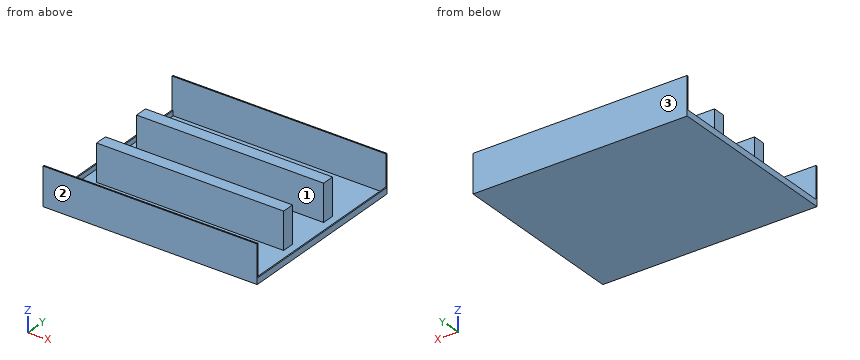
from build123d import *

# Parameters (mm, degrees)
SZKIC1_W                    = 172
SZKIC1_H                    = 144
DODANIE_WYCI_GNI_CIE1_DEPTH = 1
SZKIC1_3_W                  = 174
SZKIC1_3_H                  = 146
SZKIC1_3_W_2                = 172
SZKIC1_3_H_2                = 144
DODANIE_WYCI_GNI_CIE2_DEPTH = 5
SZKIC2_W                    = 152
SZKIC2_H                    = 10
DODANIE_WYCI_GNI_CIE4_DEPTH = 30
SZKIC4_W                    = 174
SZKIC4_H                    = 1
DODANIE_WYCI_GNI_CIE5_DEPTH = 26


with BuildPart() as part:
    # Szkic1 → Dodanie-wyciągnięcie1 (new body)
    with BuildSketch(Plane.XY):
        with Locations((86, 72)):
            Rectangle(SZKIC1_W, SZKIC1_H)
    extrude(amount=DODANIE_WYCI_GNI_CIE1_DEPTH)

    # Szkic1<3> → Dodanie-wyciągnięcie2 (add)
    with BuildSketch(Plane.XY):
        with Locations((86, 72)):
            Rectangle(SZKIC1_3_W, SZKIC1_3_H)
        with Locations((86, 72)):
            Rectangle(SZKIC1_3_W_2, SZKIC1_3_H_2, mode=Mode.SUBTRACT)
    extrude(amount=DODANIE_WYCI_GNI_CIE2_DEPTH)

    # Szkic2 → Dodanie-wyciągnięcie4 (add)
    with BuildSketch(Plane.XY.offset(1)):
        with Locations((86, 49)):
            Rectangle(SZKIC2_W, SZKIC2_H)
        with Locations((86, 94)):
            Rectangle(SZKIC2_W, SZKIC2_H)
    extrude(amount=DODANIE_WYCI_GNI_CIE4_DEPTH)

    # Szkic4 → Dodanie-wyciągnięcie5 (add)
    with BuildSketch(Plane.XY.offset(5)):
        with Locations((86, -0.5)):
            Rectangle(SZKIC4_W, SZKIC4_H)
        with Locations((86, 144.5)):
            Rectangle(SZKIC4_W, SZKIC4_H)
    extrude(amount=DODANIE_WYCI_GNI_CIE5_DEPTH)


solid = part.part
Work out the finished part from the listing and answer in its coordinate system (mm). Face numbers are marked on the shaded views. Give positions to 0.01 mm unless a question says otherwise; leave off trailing zeros. Order: outer loops, then holes, each group sorted by start corner. A loop starts at its lowest first (then second) coordinate and runs counter-clockwise, first axis right, second up. Notation, with made-up numbers: M 66.5,-6 L 86.5,-6 A26 ccw 86.5,27 Z; hole C -33.5,-26.5 d6. An arc over 180 degrees is marked long. Return JSON: item names as keys, results as strings.
Q1. Find section A-A, the plane z = 8.5. Write down the section's boundary in (x, y), and give its area (3 significant figures).
Answer below:
{"outline": "M -1,-1 L 173,-1 L 173,0 L -1,0 Z; M -1,144 L 173,144 L 173,145 L -1,145 Z; M 10,44 L 162,44 L 162,54 L 10,54 Z; M 10,89 L 162,89 L 162,99 L 10,99 Z", "area": "3,390 mm^2"}
Q2. The mould has two halves that part along Y. Classify the marked faces 1, 2 and 3: pulls with the +Y half, pulls with the -Y half, needs draft (parallel to the pull), parting line crosses it, or undercut.
Answer below:
{"face 1": "undercut", "face 2": "pulls with the -Y half", "face 3": "pulls with the +Y half"}
Q3. Find section C-C, the plane x = 147.5. Write down the section's boundary in (y, z), and give its area (3 significant figures).
Answer below:
{"outline": "M -1,0 L 145,0 L 145,31 L 144,31 L 144,1 L 99,1 L 99,31 L 89,31 L 89,1 L 54,1 L 54,31 L 44,31 L 44,1 L 0,1 L 0,31 L -1,31 Z", "area": "806 mm^2"}
Q4. Each of these flat-tipped pins is pushed along its axis until it touches: pin 1 (8 mm diameter, centred on y = 47, z = 13.5, fed in from -X); pin 2 (0.8 mm diameter, centred on x = 172.5, y = 53, fed in from +Z); pin 3 (5 mm diameter, centred on y = 47.5, z = 9.5, fed in from +X). Where does it stop, or does it pass through?
Answer below:
{"pin 1": "stops at x = 10", "pin 2": "stops at z = 5", "pin 3": "stops at x = 162"}
Q5. Find the intervals of material crossed by line 1 along Y through (x, z) = (118.5, 26); line 2 along X through (y, z) = (63, 4.5); line 3 along Y through (x, z) = (163, 27.5), in increasing order. Write a range as [from, to].
Answer below:
{"line 1": "y = [-1, 0], [44, 54], [89, 99], [144, 145]", "line 2": "x = [-1, 0], [172, 173]", "line 3": "y = [-1, 0], [144, 145]"}
Q6. Find section D-D, the plane y = 48. Write down the section's boundary in (x, z), and give its area (3 significant figures).
Answer below:
{"outline": "M -1,0 L 173,0 L 173,5 L 172,5 L 172,1 L 162,1 L 162,31 L 10,31 L 10,1 L 0,1 L 0,5 L -1,5 Z", "area": "4,740 mm^2"}
Q7. Find section B-B, the plane y = 30.5. Write down the section's boundary in (x, z), and give its area (3 significant figures).
Answer below:
{"outline": "M -1,0 L 173,0 L 173,5 L 172,5 L 172,1 L 0,1 L 0,5 L -1,5 Z", "area": "182 mm^2"}
